from build123d import *

# Parameters (mm, degrees)
SKETCH1_W                 = 330.2
SKETCH1_H                 = 50.8
BOSS_EXTRUDE1_DEPTH       = 25.4
SKETCH2_W                 = 20.32
SKETCH2_H                 = 45.72
CUT_EXTRUDE1_DEPTH        = 331.2
F_6_CLEARANCE_HOLE1_D     = 4.1402
F_6_CLEARANCE_HOLE1_DEPTH = 50.8
F_6_CLEARANCE_HOLE2_D     = 4.1402
F_6_CLEARANCE_HOLE2_DEPTH = 50.8
FILLET1_R                 = 0.5
FILLET2_R                 = 2.54


with BuildPart() as part:
    # Sketch1 → Boss-Extrude1 (new body)
    with BuildSketch(Plane(origin=(12.7, 0, 0), x_dir=(0, 0, -1), z_dir=(1, 0, 0))):
        Rectangle(SKETCH1_W, SKETCH1_H)
    extrude(amount=-BOSS_EXTRUDE1_DEPTH)

    # Sketch2 → Cut-Extrude1 (cut, through all)
    with BuildSketch(Plane(origin=(0, 0, -165.1), x_dir=(-1, 0, 0), z_dir=(0, 0, -1))):
        Rectangle(SKETCH2_W, SKETCH2_H)
    extrude(amount=-CUT_EXTRUDE1_DEPTH, mode=Mode.SUBTRACT)

    # #6 Clearance Hole1
    with Locations(Plane(origin=(0, -25.4, 0), x_dir=(-1, 0, 0), z_dir=(0, -1, 0))):
        with Locations((0, 711.2), (0, 736.6), (0, 685.8), (0, 660.4), (0, 635), (0, 609.6), (0, 584.2), (0, 558.8), (0, 533.4), (0, 508), (0, 482.6), (0, 457.2), (0, 431.8), (0, 406.4), (0, 381), (0, 355.6), (0, 330.2), (0, 304.8), (0, 279.4), (0, 254), (0, 228.6), (0, 203.2), (0, 177.8), (0, 152.4), (0, 127), (0, 101.6), (0, 76.2), (0, 50.8), (0, 25.4), (0, 0), (0, -25.4), (0, -50.8), (0, -76.2), (0, -101.6), (0, -127), (0, -152.4), (0, -177.8), (0, -203.2), (0, -228.6), (0, -254), (0, -279.4), (0, -304.8), (0, -330.2), (0, -355.6), (0, -381), (0, -406.4), (0, -431.8), (0, -457.2), (0, -482.6), (0, -508), (0, -533.4), (0, -558.8), (0, -584.2), (0, -609.6), (0, -635), (0, -660.4), (0, -685.8), (0, -711.2), (0, -736.6)):
            Hole(F_6_CLEARANCE_HOLE1_D / 2, depth=F_6_CLEARANCE_HOLE1_DEPTH)

    # #6 Clearance Hole2
    with Locations(Plane(origin=(0, 25.4, 0), x_dir=(1, 0, 0), z_dir=(0, 1, 0))):
        with Locations((0, 711.2), (0, 736.6), (0, 685.8), (0, 660.4), (0, 635), (0, 609.6), (0, 584.2), (0, 558.8), (0, 533.4), (0, 508), (0, 482.6), (0, 457.2), (0, 431.8), (0, 406.4), (0, 381), (0, 355.6), (0, 330.2), (0, 304.8), (0, 279.4), (0, 254), (0, 228.6), (0, 203.2), (0, 177.8), (0, 152.4), (0, 127), (0, 101.6), (0, 76.2), (0, 50.8), (0, 25.4), (0, 0), (0, -25.4), (0, -50.8), (0, -76.2), (0, -101.6), (0, -127), (0, -152.4), (0, -177.8), (0, -203.2), (0, -228.6), (0, -254), (0, -279.4), (0, -304.8), (0, -330.2), (0, -355.6), (0, -381), (0, -406.4), (0, -431.8), (0, -457.2), (0, -482.6), (0, -508), (0, -533.4), (0, -558.8), (0, -584.2), (0, -609.6), (0, -635), (0, -660.4), (0, -685.8), (0, -711.2), (0, -736.6)):
            Hole(F_6_CLEARANCE_HOLE2_D / 2, depth=F_6_CLEARANCE_HOLE2_DEPTH)

    # Fillet1
    fillet1_edges = [part.edges().sort_by_distance(p)[0] for p in [
        (-10.16, -22.86, 0),
        (10.16, -22.86, 0),
        (10.16, 22.86, 0),
        (-10.16, 22.86, 0),
    ]]
    fillet(fillet1_edges, radius=FILLET1_R)

    # Fillet2
    fillet2_edges = [part.edges().sort_by_distance(p)[0] for p in [
        (-12.7, 25.4, 0),
        (-12.7, -25.4, 0),
        (12.7, 25.4, 0),
        (12.7, -25.4, 0),
    ]]
    fillet(fillet2_edges, radius=FILLET2_R)


solid = part.part
CAD build for the part. Positions are in the model's coordinates, mm. A direction names the side the tool comes from. Round coordinates to 2 decimals unless told otherwise and drop trailing zeros. Write each loop counter-clockwise with the first axis right and the second up, starting at its lowest first coordinate (ties: lowest second). Pieces come first, ordered by that corner, then holes. Notation, with made-up numbers: M 5.5,64 L 22.5,64 A25 cw 22.5,95 Z; hole C -28,67 d7. An arc over 180 degrees is marked long. Use a Markdown table: item, result. Add a question column.
1. Slice it at A-A on y = 0.5. Give the cut face in (x, z), then the cut area to 3 significant figures.
2. 3-axis set-ups, long thin cutter, end or side, ignore diameter. For faces 4 (the face through (-10.16, 0, -2)), 5 (the face through (-12.7, 0, 2)): which of +Z, -Z, +X, -X, +Y, -Y reach the whole face in a straight line?
3. Drill centre lines: probe 1 along Y at (x, z) = (-7.5, 115); probe 2 along X at (y, z) = (-10.5, 69.5); probe 3 along X at (y, z) = (-22.5, 84.5). Where is each one in solid material? Low to high.
4. Slice it at B-B on z = -45.5. Give the cut face in (x, y).
5. Pull direction X, two halves, no side cores. Call faces 1 (the face through (0.1, -22.86, -2.3)), 2 (the face through (10.4, -2, -165.1)), 3 (the face through (12.7, 0, 2)): released by +X, released by -X, zero draft, split by the parting line, or undercut.
Reply:
| question | item | result |
|---|---|---|
| 1 | outline | M -12.7,-165.1 L -10.16,-165.1 L -10.16,165.1 L -12.7,165.1 Z; M 10.16,-165.1 L 12.7,-165.1 L 12.7,165.1 L 10.16,165.1 Z |
| 1 | area | 1,680 mm^2 |
| 2 | face 4 | +Z, -Z |
| 2 | face 5 | +Z, -Z, -X, +Y, -Y |
| 3 | probe 1 | y = -25.4 to -22.86, 22.86 to 25.4 |
| 3 | probe 2 | x = -12.7 to -10.16, 10.16 to 12.7 |
| 3 | probe 3 | x = -12.7 to -10.14, 10.14 to 12.7 |
| 4 | outline | M -12.7,-22.86 A2.54 ccw -10.16,-25.4 L 10.16,-25.4 A2.54 ccw 12.7,-22.86 L 12.7,22.86 A2.54 ccw 10.16,25.4 L -10.16,25.4 A2.54 ccw -12.7,22.86 Z; hole M -10.16,-22.36 A0.5 ccw -9.66,-22.86 L 9.66,-22.86 A0.5 ccw 10.16,-22.36 L 10.16,22.36 A0.5 ccw 9.66,22.86 L -9.66,22.86 A0.5 ccw -10.16,22.36 Z |
| 5 | face 1 | undercut |
| 5 | face 2 | zero draft |
| 5 | face 3 | released by +X |
